Geometry: final body of the model. Coordinates: model frame, mm. A direction names the side the tool comes from. Give positions to 0.01 mm unless a question says otherwise; leave off trailing zeros. Order: outer loops, then holes, each group sorted by start corner. A loop starts at its lowest first (then second) coordinate and runs counter-clockwise, first axis right, second up. Notation, with made-up numbers: (-1, 30.5) -> (4, 30.5) arc R25 ccw to (4, 45.5) -> close; hole circle Ø6 at (-35.5, 8.5). An arc over 180 degrees is marked (long way). One line per question, with ' | ' between items.
from build123d import *

# Parameters (mm, degrees)
SKETCH_1_W          = 56
SKETCH_1_H          = 25
EXTRUDE_1_DEPTH     = 2
EXTRUDE_2_DEPTH     = 2
SKETCH_3_R          = 4
SKETCH_3_R_2        = 1
CUT_EXTRUDE_1_DEPTH = 105
SKETCH_4_R          = 1.5
CUT_EXTRUDE_2_DEPTH = 105
SKETCH_5_R          = 1.5
CUT_EXTRUDE_3_DEPTH = 105
SKETCH_6_R          = 1.5
SKETCH_6_R_2        = 4
CUT_EXTRUDE_5_DEPTH = 105
CUT_EXTRUDE_6_DEPTH = 84.41891632


with BuildPart() as part:
    # 草图1 → 凸台-拉伸1 (new body)
    with BuildSketch(Plane(origin=(0, 0, 0), x_dir=(1, 0, 0), z_dir=(0, 1, 0))):
        with Locations((14.16, -0.793333333)):
            Rectangle(SKETCH_1_W, SKETCH_1_H)
    extrude(amount=EXTRUDE_1_DEPTH)

    # 草图2 → 凸台-拉伸2 (add)
    with BuildSketch(Plane(origin=(42.16, 0, 0), x_dir=(0, 0, -1), z_dir=(1, 0, 0))):
        with BuildLine():
            Line((-13.293333333, 2), (-13.293333333, 55))
            ThreePointArc((-13.293333333, 55), (-0.793333333, 67.5), (11.706666667, 55))
            Line((11.706666667, 55), (11.706666667, 2))
            Line((11.706666667, 2), (-13.293333333, 2))
        make_face()
    extrude_2 = extrude(amount=-EXTRUDE_2_DEPTH)

    # 镜向1: 凸台-拉伸2 across plane
    add(extrude_2.mirror(Plane.ZY.offset(-14.16)))

    # 草图3 → 切除-拉伸1 (cut)
    with BuildSketch(Plane(origin=(42.16, 0, 0), x_dir=(0, 0, -1), z_dir=(1, 0, 0))):
        with Locations((-0.793333333, 55)):
            Circle(SKETCH_3_R)
        with Locations((-0.793333333, 62)):
            Circle(SKETCH_3_R_2)
        with Locations((4.156414135, 59.949747468)):
            Circle(SKETCH_3_R_2)
        with Locations((6.206666667, 55)):
            Circle(SKETCH_3_R_2)
        with Locations((4.156414135, 50.050252532)):
            Circle(SKETCH_3_R_2)
        with Locations((-0.793333333, 48)):
            Circle(SKETCH_3_R_2)
        with Locations((-5.743080802, 50.050252532)):
            Circle(SKETCH_3_R_2)
        with Locations((-7.793333333, 55)):
            Circle(SKETCH_3_R_2)
        with Locations((-5.743080802, 59.949747468)):
            Circle(SKETCH_3_R_2)
    extrude(amount=-CUT_EXTRUDE_1_DEPTH, mode=Mode.SUBTRACT)

    # 草图4 → 切除-拉伸2 (cut)
    with BuildSketch(Plane(origin=(42.16, 0, 0), x_dir=(0, 0, -1), z_dir=(1, 0, 0))):
        with Locations((-0.793333333, 17.5)):
            Circle(SKETCH_4_R)
        with Locations((-0.793333333, 35)):
            Circle(SKETCH_4_R)
    extrude(amount=-CUT_EXTRUDE_2_DEPTH, mode=Mode.SUBTRACT)

    # 草图5 → 切除-拉伸3 (cut)
    with BuildSketch(Plane(origin=(0, 2, 0), x_dir=(1, 0, 0), z_dir=(0, 1, 0))):
        with Locations(Location((32.16, -0.793333333, 0), (0, 0, 270))):
            Circle(SKETCH_5_R)
        with BuildLine():
            ThreePointArc((-3.84, 0.706666667), (-5.34, -0.793333333), (-3.84, -2.293333333))
            Line((-3.84, -2.293333333), (-3.84, 0.706666667))
        make_face()
        with BuildLine():
            Line((-3.84, 0.706666667), (-3.84, -2.293333333))
            ThreePointArc((-3.84, -2.293333333), (-2.779339828, -1.853993505), (-2.34, -0.793333333))
            ThreePointArc((-2.34, -0.793333333), (-2.779339828, 0.267326838), (-3.84, 0.706666667))
        make_face()
    extrude(amount=-CUT_EXTRUDE_3_DEPTH, mode=Mode.SUBTRACT)

    # 草图6 → 切除-拉伸5 (cut)
    with BuildSketch(Plane(origin=(0, 2, 0), x_dir=(1, 0, 0), z_dir=(0, 1, 0))):
        with Locations(Location((14.16, -7.793333333, 0), (0, 0, 270))):
            Circle(SKETCH_6_R)
        with Locations(Location((9.210252532, -5.743080802, 0), (0, 0, 270))):
            Circle(SKETCH_6_R)
        with Locations(Location((7.16, -0.793333333, 0), (0, 0, 270))):
            Circle(SKETCH_6_R)
        with Locations(Location((9.210252532, 4.156414135, 0), (0, 0, 270))):
            Circle(SKETCH_6_R)
        with Locations(Location((14.16, 6.206666667, 0), (0, 0, 270))):
            Circle(SKETCH_6_R)
        with Locations(Location((19.109747468, 4.156414135, 0), (0, 0, 270))):
            Circle(SKETCH_6_R)
        with Locations(Location((21.16, -0.793333333, 0), (0, 0, 270))):
            Circle(SKETCH_6_R)
        with Locations(Location((19.109747468, -5.743080802, 0), (0, 0, 270))):
            Circle(SKETCH_6_R)
        with Locations(Location((14.16, -0.793333333, 0), (0, 0, 270))):
            Circle(SKETCH_6_R_2)
    extrude(amount=-CUT_EXTRUDE_5_DEPTH, mode=Mode.SUBTRACT)

    # 草图7 → 切除-拉伸6 (cut, through all)
    with BuildSketch(Plane.XY.offset(13.293333333)):
        with BuildLine():
            Line((-13.84, 0), (-11.84, 0))
            ThreePointArc((-11.84, 0), (-13.254213562, 0.585786438), (-13.84, 2))
            Line((-13.84, 2), (-13.84, 0))
        make_face()
        with BuildLine():
            ThreePointArc((42.16, 2), (41.574213562, 0.585786438), (40.16, 0))
            Line((40.16, 0), (42.16, 0))
            Line((42.16, 0), (42.16, 2))
        make_face()
    extrude(amount=-CUT_EXTRUDE_6_DEPTH, mode=Mode.SUBTRACT)


solid = part.part
1) Section A-A on x = 32.16. Return loops of the section in (y, z), plus the area to 3 significant figures.
Check result:
outline: (0, -11.71) -> (2, -11.71) -> (2, -0.71) -> (0, -0.71) -> close; (0, 2.29) -> (2, 2.29) -> (2, 13.29) -> (0, 13.29) -> close | area: 44.0 mm^2
2) Material intervals for probe 1 along X at (y, z) = (47, 2); probe 2 along Y at (x, z) = (37, 0.5), sorted ascending. Write a range as from..to.
Check result:
probe 1: x = -13.84..-11.84, 40.16..42.16 | probe 2: y = 0..2
3) Contact query for flat-ended pins moving along their axis: pin 1 Ø3.5 at (x, z) = (21.16, 0.79) entering from -Y; pin 2 Ø1.8 at (x, z) = (9.21, -4.16) entering from -Y; pin 3 Ø7.5 at (x, z) = (21.5, -4) entering from +Y. Output: stop coordinate, or through.
Check result:
pin 1: stops at y = 0 | pin 2: passes through | pin 3: stops at y = 2
4) Pull-direction query (X, two-part tool) for faces 3 (the cylindrical face through (12.696, 1.014, -6.532)), 4 (the flat face through (42.16, 35, 3)), 5 (the cylindrical face through (-12.826, 33.536, 1.119)); classes: +X half, -X half, draft (parallel to the pull), parting line (faces both ways), or undercut.
Check result:
face 3: undercut | face 4: +X half | face 5: draft
5) Set-up query: faces 1 (the cylindrical face through (19.696, 1.014, 0.468)), 2 (the flat face through (14, 2, 6)). Return all of +Z, -Z, +X, -X, +Y, -Y with unobstructed straight access to the full face (end or side cutting, diameter ignored); none if empty.
Check result:
face 1: +Y, -Y | face 2: +Z, -Z, +Y
6) Section D-D on z = 8. Return loops of the section in (x, y).
Check result:
outline: (-13.84, 2) arc R2 ccw to (-11.84, 0) -> (12.67, 0) -> (12.67, 2) -> (-11.84, 2) -> (-11.84, 54.02) -> (-13.84, 54.02) -> close; (-13.84, 55.98) -> (-11.84, 55.98) -> (-11.84, 65.21) -> (-13.84, 65.21) -> close; (15.65, 0) -> (40.16, 0) arc R2 ccw to (42.16, 2) -> (42.16, 54.02) -> (40.16, 54.02) -> (40.16, 2) -> (15.65, 2) -> close; (40.16, 55.98) -> (42.16, 55.98) -> (42.16, 65.21) -> (40.16, 65.21) -> close
7) Section C-C on y = 48. Return loops of the section in (x, z).
Check result:
outline: (-13.84, -11.71) -> (-11.84, -11.71) -> (-11.84, -0.21) -> (-13.84, -0.21) -> close; (-13.84, 1.79) -> (-11.84, 1.79) -> (-11.84, 13.29) -> (-13.84, 13.29) -> close; (40.16, -11.71) -> (42.16, -11.71) -> (42.16, -0.21) -> (40.16, -0.21) -> close; (40.16, 1.79) -> (42.16, 1.79) -> (42.16, 13.29) -> (40.16, 13.29) -> close
8) Section B-B on y = 4. Return loops of the section in (x, z), plus the area to 3 significant figures.
Check result:
outline: (-13.84, -11.71) -> (-11.84, -11.71) -> (-11.84, 13.29) -> (-13.84, 13.29) -> close; (40.16, -11.71) -> (42.16, -11.71) -> (42.16, 13.29) -> (40.16, 13.29) -> close | area: 100 mm^2
